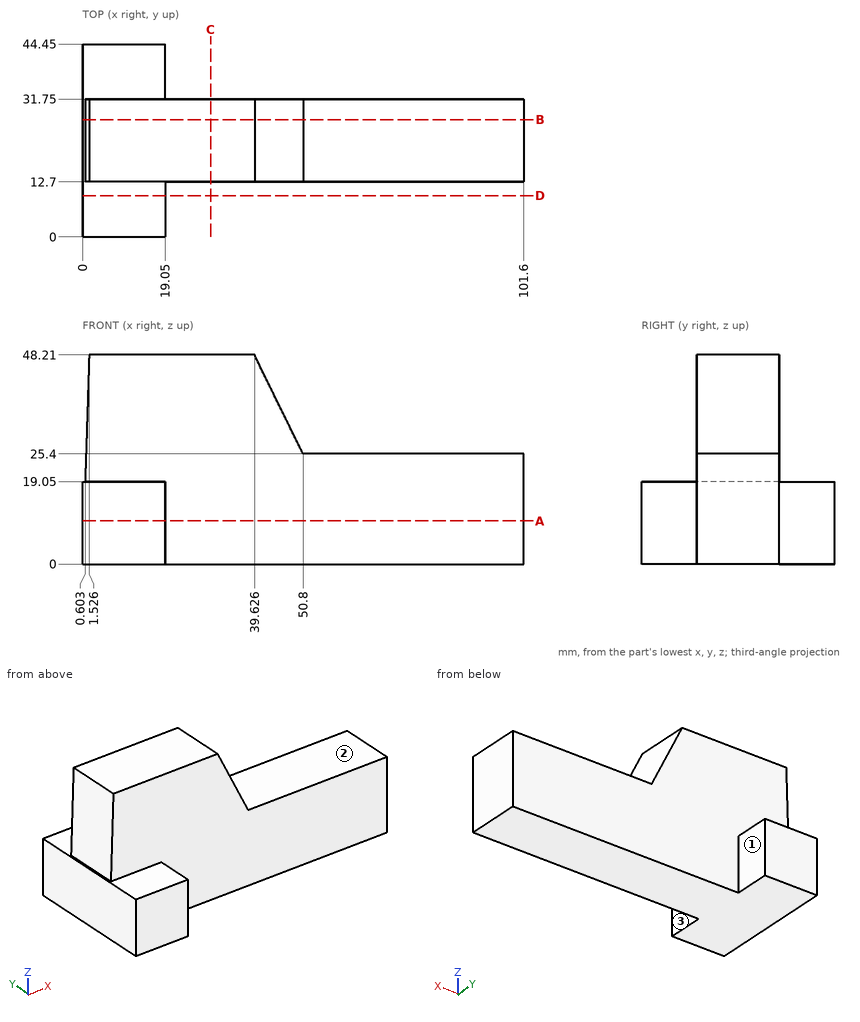
Drawing for the job (mm, zero at the part's lowest x, y, z). A direction names the side the tool comes from. Give positions to 0.01 mm unless a question says otherwise; leave off trailing zeros. Order: outer loops, then holes, each group sorted by start corner. A loop starts at its lowest first (then second) coordinate and runs counter-clockwise, first axis right, second up. Notation, with made-up numbers: (-1, 54.5) - (25, 54.5) arc R5 ccw to (25, 59.5) - close; hole circle Ø11 at (70.25, 64.5). An arc over 180 degrees is marked (long way). Write item = value, one per line. Start each with the question number.
1. Probe line 1 along Y through (x, z) = (74.5, 25); line 2 along Z through (x, y) = (87, 23); line 3 along X through (y, z) = (37.5, 6). List the from-to ranges inside material, lowest first.
2. Cut at D-D, the plane y = 9.5. List the corners of the cut face in (x, z).
3. Cut at C-C, the plane x = 29.5. List the corners of the cut face in (y, z).
4. Which spindle directions (+Z, -Z, +X, -X, +Y, -Y) get a long thin tool onto all of the face, cutting with end or side? Do the marked faces 1, 2 and 3. Say none if no direction does.
5. Cut at B-B, the plane y = 27. List the corners of the cut face in (x, z), and give its area (3 significant figures).
6. Cut at A-A, the plane z = 10. List the corners of the cut face in (x, y), and give its area (3 significant figures).
7. Drop flat-ended pins along their axis: P1, Ø4, axis at y = 38.5, z = 13, coming from the +X side; P2, Ø5, axis at x = 80, y = 20.5, coming from the +Z side; P3, Ø4, axis at x = 11.5, z = 42.5, coming from the -Y side. Give the stop position or say it passes through.
Taken from the geometry:
q1.line_1 = 12.7 to 31.75
q1.line_2 = 0 to 25.4
q1.line_3 = 0 to 19.05
q2.outline = (0, 0) - (19.05, 0) - (19.05, 19.05) - (0, 19.05) - close
q3.outline = (12.7, 0) - (31.75, 0) - (31.75, 48.21) - (12.7, 48.21) - close
q4.face_1 = +Z, -Z, +X, +Y
q4.face_2 = +Z, +X, +Y, -Y
q4.face_3 = +Z, -Z, +X, -Y
q5.outline = (0, 0) - (101.6, 0) - (101.6, 25.4) - (50.8, 25.4) - (39.63, 48.21) - (1.53, 48.21) - (0.6, 19.05) - (0, 19.05) - close
q5.area = 3,580 mm²
q6.outline = (0, 0) - (19.05, 0) - (19.05, 12.7) - (101.6, 12.7) - (101.6, 31.75) - (19.05, 31.75) - (19.05, 44.45) - (0, 44.45) - close
q6.area = 2,420 mm²
q7.P1 = 19.05
q7.P2 = 25.4
q7.P3 = 12.7
